Check sheet for the modelled part. Datum: model origin and axes. Units: mm. Face numbers are marked on the shaded views. Coordinates: 2 decimals unless noted, no trailing zeros. Loops run counter-clockwise (first coordinate to the right, second up) from the corner with the lowest first, then second, coordinate; pieces in that order, holes last.
```python
from build123d import *

# Parameters (mm, degrees)
SKETCH1_W               = 254
SKETCH1_H               = 254
BOSS_EXTRUDE1_DEPTH     = 25.4
F_10_CLEARANCE_HOLE1_D  = 5.1054
F_1_1_115_DOWEL_HOLE1_D = 28.321


with BuildPart() as part:
    # Sketch1 → Boss-Extrude1 (new body)
    with BuildSketch(Plane(origin=(0, 0, 0), x_dir=(1, 0, 0), z_dir=(0, 1, 0))):
        Rectangle(SKETCH1_W, SKETCH1_H)
    extrude(amount=BOSS_EXTRUDE1_DEPTH)

    # #10 Clearance Hole1 (through all)
    with Locations(Plane(origin=(0, 0, 0), x_dir=(-1, 0, 0), z_dir=(0, -1, 0))):
        with Locations((-61.414487758, 62.639487758), (-97.335512242, 98.560512242), (-61.875, 98.1), (-96.875, 63.1)):
            Hole(F_10_CLEARANCE_HOLE1_D / 2)

    # 1 (1.115) Dowel Hole1 (through all)
    with Locations(Plane(origin=(0, 0, 0), x_dir=(-1, 0, 0), z_dir=(0, -1, 0))):
        with Locations((-79.375, 80.6)):
            Hole(F_1_1_115_DOWEL_HOLE1_D / 2)


solid = part.part
```
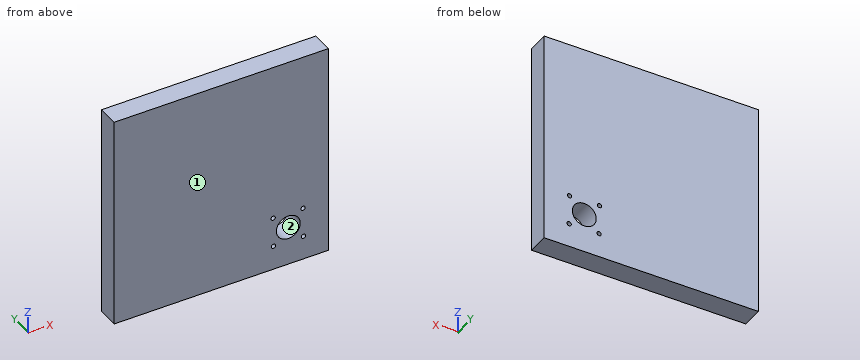
1) Section check A-A on x = 88.5. Enter the section's corners in (y, z).
Answer sheet:
outline: (0, -127) - (25.4, -127) - (25.4, -91.43) - (0, -91.43) - close; (0, -69.77) - (25.4, -69.77) - (25.4, 127) - (0, 127) - close
2) Scan lines: line 1 (X direction, y = 11.5, z = -63.1); line 2 (X direction, y = 5.75, z = -98.1); line 3 (Z direction, x = 78, y = 6.25). Record each from-to range of solid material in increasing order.
Answer sheet:
line 1: x = -127 to 58.9, 63.93 to 94.32, 99.43 to 127
line 2: x = -127 to 59.32, 64.43 to 94.82, 99.85 to 127
line 3: z = -127 to -94.69, -66.51 to 127
3) Depth check by flat-ended pin: pin 1 (6.5 mm diameter, centred on x = 96.875, z = -63.1, fed in from -Y); pin 2 (4 mm diameter, centred on x = 97.34, z = -98.56, fed in from +Y). Enter the tip coordinate at first touch or a pass-through.
Answer sheet:
pin 1: stops at y = 0
pin 2: passes through
4) Mould release check, pull along Z, two halves, no side actions. Record for the marked faces 1 and 2: +Z half, -Z half, draft (parallel to the pull), parting line (faces both ways), or undercut.
Answer sheet:
face 1: draft
face 2: undercut
5) Section check B-B on z = -80.6. Enter the section's corners in (x, y).
Answer sheet:
outline: (-127, 0) - (65.21, 0) - (65.21, 25.4) - (-127, 25.4) - close; (93.54, 0) - (127, 0) - (127, 25.4) - (93.54, 25.4) - close
